Verification items for this drawing (mm, ordinates from the low corner). A direction names the side the tool comes from. Give positions to 0.01 mm unless a question says otherwise; leave off trailing zeros. Order: outer loops, then holes, each group sorted by start corner. A loop starts at its lowest first (then second) coordinate and runs counter-clockwise, first axis right, second up. Notation, with made-up numbers: M 83,-8 L 89,-8 A4 ccw 89,-3 Z; hole C -18,77 d3. An arc over 180 degrees is marked long. Answer as a JSON object with one key per item and string values.
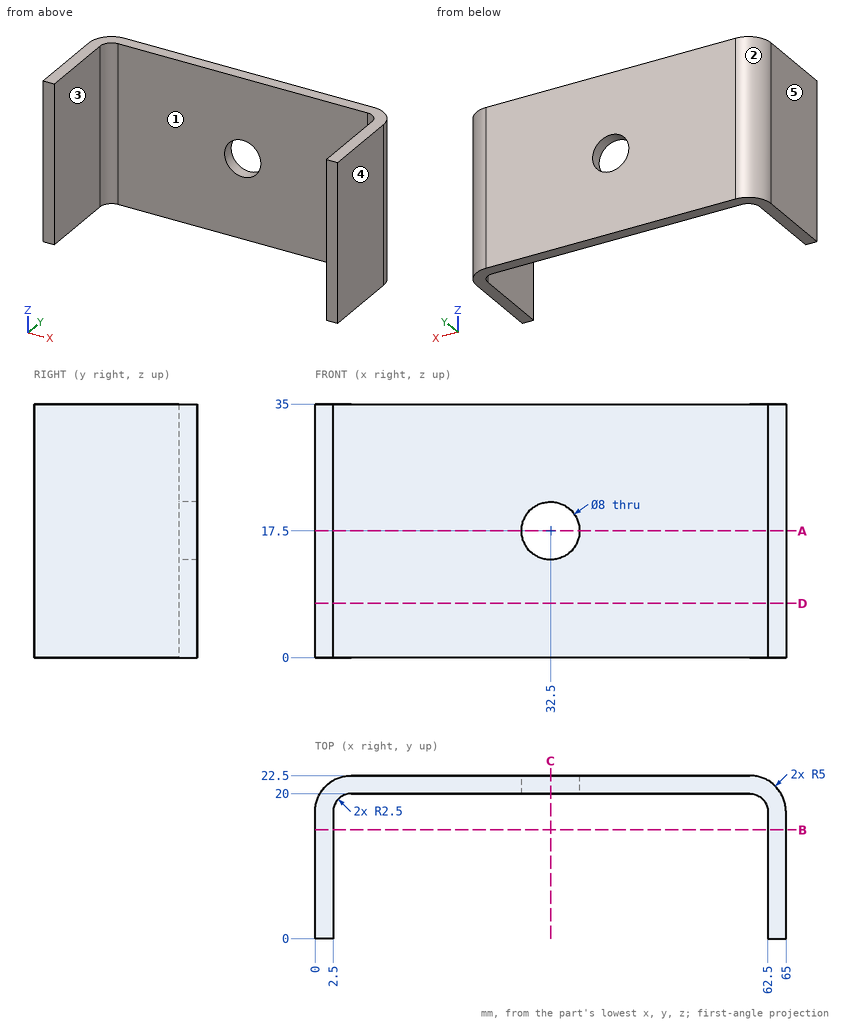
Q1. Section check A-A on z = 17.5. Record the cut outline in (x, y), then the cut area to 3 significant figures.
Resolved:
{"outline": "M 0,0 L 2.5,0 L 2.5,17.5 A2.5 cw 5,20 L 28.5,20 L 28.5,22.5 L 5,22.5 A5 ccw 0,17.5 Z; M 36.5,20 L 60,20 A2.5 cw 62.5,17.5 L 62.5,0 L 65,0 L 65,17.5 A5 ccw 60,22.5 L 36.5,22.5 Z", "area": "234 mm²"}
Q2. Section check D-D on z = 7.5. Record the cut outline in (x, y).
Resolved:
{"outline": "M 0,0 L 2.5,0 L 2.5,17.5 A2.5 cw 5,20 L 60,20 A2.5 cw 62.5,17.5 L 62.5,0 L 65,0 L 65,17.5 A5 ccw 60,22.5 L 5,22.5 A5 ccw 0,17.5 Z"}
Q3. Section check C-C on x = 32.5. Record the cut outline in (y, z), then the cut area to 3 significant figures.
Resolved:
{"outline": "M 20,0 L 22.5,0 L 22.5,13.5 L 20,13.5 Z; M 20,21.5 L 22.5,21.5 L 22.5,35 L 20,35 Z", "area": "67.5 mm²"}
Q4. Gauge pin test, flat end, axial feed: pin 1 Ø6 at (x, z) = (38, 28) entering from -Y. Record the tip position at first contact, or that the pin passes through.
Resolved:
{"pin 1": "stops at y = 20"}
Q5. Material ranges on L1, parallel to X at y = 2.75, z = 8; L2, parallel to Z at x = 32.5, y = 21.1; L3, parallel to Y at x = 12, z = 30, recorded low to high.
Resolved:
{"L1": "x = 0 to 2.5, 62.5 to 65", "L2": "z = 0 to 13.5, 21.5 to 35", "L3": "y = 20 to 22.5"}
Q6. Release check for a two-part mould opening along X. For the marked faces 3, 4 and 5 record: +X half, -X half, draft (parallel to the pull), parting line (faces both ways), or undercut.
Resolved:
{"face 3": "undercut", "face 4": "+X half", "face 5": "-X half"}
Q7. Section check B-B on y = 15. Record the cut outline in (x, z), then the cut area to 3 significant figures.
Resolved:
{"outline": "M 0,0 L 2.5,0 L 2.5,35 L 0,35 Z; M 62.5,0 L 65,0 L 65,35 L 62.5,35 Z", "area": "175 mm²"}
Q8. Tool access check on the marked faces 1 and 2. Record the directions out of +Z, -Z, +X, -X, +Y, -Y that give a thin tool (end or side, any length) a straight path to the whole face; none if there is none.
Resolved:
{"face 1": "+Z, -Z, -Y", "face 2": "+Z, -Z, -X, +Y"}
